from build123d import *

# Parameters (mm, degrees)
MAIN_BOARD_W          = 1000
MAIN_BOARD_H          = 750
MAINBOARD_DEPTH       = 20
CUT_EXTRUDE9_REACH    = 627.32
SKETCH5_R             = 10
SKETCH5_8_R           = 110
SKETCH5_8_R_2         = 105
CUT_EXTRUDE10_DEPTH   = 15
LPATTERN1_START       = 5
LPATTERN1_OUTLINE_R   = 110
LPATTERN1_OUTLINE_R_2 = 105
LPATTERN1_DEPTH       = 15


# Read off the part's stored shape, not the designer's step: LPattern1
with BuildPart() as part:
    # Main Board → MainBoard (new body)
    with BuildSketch(Plane(origin=(0, 0, 0), x_dir=(0, 0, -1), z_dir=(1, 0, 0))):
        Rectangle(MAIN_BOARD_W, MAIN_BOARD_H)
    extrude(amount=MAINBOARD_DEPTH)

    # Sketch5 → Cut-Extrude9 (cut, up to next)
    with BuildSketch(Plane(origin=(20, 0, 0), x_dir=(0, 0, -1), z_dir=(1, 0, 0)), mode=Mode.PRIVATE) as cut_extrude9_sk1:
        with Locations((-250, 125)):
            Circle(SKETCH5_R)
    cut_extrude9_tool1 = extrude(cut_extrude9_sk1.sketch, amount=-CUT_EXTRUDE9_REACH, mode=Mode.PRIVATE) & part.part
    add(cut_extrude9_tool1.solids().sort_by_distance((20, 125, 250))[0], mode=Mode.SUBTRACT)

    # Sketch5<8> → Cut-Extrude10 (cut)
    with BuildSketch(Plane(origin=(20, 0, 0), x_dir=(0, 0, -1), z_dir=(1, 0, 0))):
        with Locations((-250, 125)):
            Circle(SKETCH5_8_R)
        with Locations((-250, 125)):
            Circle(SKETCH5_8_R_2, mode=Mode.SUBTRACT)
    extrude(amount=-CUT_EXTRUDE10_DEPTH, mode=Mode.SUBTRACT)

    # LPattern1 outline → LPattern1 (cut)
    # profile 1 of 4: a face of its own
    with BuildSketch(Plane.YZ.offset(LPATTERN1_START)):
        with Locations((-91, 125)):
            Circle(LPATTERN1_OUTLINE_R)
        with Locations((-91, 125)):
            Circle(LPATTERN1_OUTLINE_R_2, mode=Mode.SUBTRACT)
    # profile 2 of 4: a face of its own
    with BuildSketch(Plane.YZ.offset(LPATTERN1_START)):
        with Locations((125, -250)):
            Circle(LPATTERN1_OUTLINE_R)
        with Locations((125, -250)):
            Circle(LPATTERN1_OUTLINE_R_2, mode=Mode.SUBTRACT)
    # profile 3 of 4: a face of its own
    with BuildSketch(Plane.YZ.offset(LPATTERN1_START)):
        with Locations((125, 0)):
            Circle(LPATTERN1_OUTLINE_R)
        with Locations((125, 0)):
            Circle(LPATTERN1_OUTLINE_R_2, mode=Mode.SUBTRACT)
    # profile 4 of 4: a face of its own
    with BuildSketch(Plane.YZ.offset(LPATTERN1_START)):
        with Locations((-91, -125)):
            Circle(LPATTERN1_OUTLINE_R)
        with Locations((-91, -125)):
            Circle(LPATTERN1_OUTLINE_R_2, mode=Mode.SUBTRACT)
    extrude(amount=LPATTERN1_DEPTH, mode=Mode.SUBTRACT)


solid = part.part
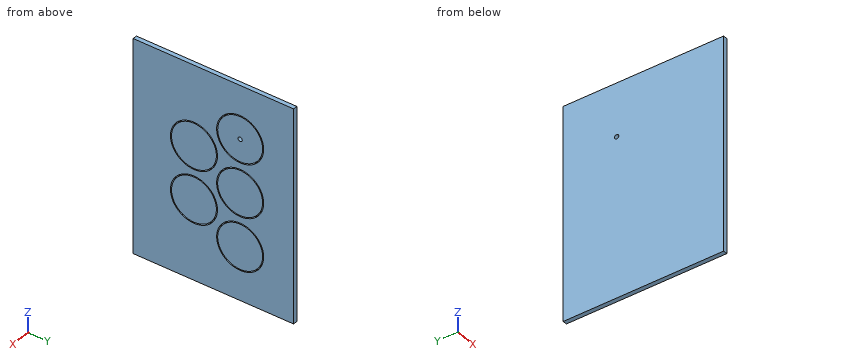
The listing builds one solid part. Answer for the finished solid, in the listing's coordinates (mm). Coordinates: 2 decimals unless noted, no trailing zeros. Write each loop counter-clockwise with the first axis right and the second up, starting at its lowest first coordinate (ties: lowest second). Pieces come first, ordered by that corner, then holes. Notation, with made-up numbers: (68, -30.5) -> (114, -30.5) arc R24 ccw to (114, -14.5) -> close; hole circle Ø2 at (3, 56). An arc over 180 degrees is marked (long way). One line per question, with ' | ' between items.
1. Section A-A (x = 14.25) is taken. State how many separate pieces and enclosed holes the cut face has, and give its area (3 significant figures).
Verdict:
separate pieces: 6 | enclosed holes: 6 | area: 733,000 mm^2
2. Straight lines are drawn through the part: line 1 (Y direction, x = 15.25, z = 250); line 2 (Z direction, x = 11.5, y = -91); line 3 (Y direction, x = 18.75, z = 219.5). For each, find the intervals that lie inside material, in ascending order.
Verdict:
line 1: y = -375 to 15, 20 to 115, 135 to 230, 235 to 375 | line 2: z = -500 to -235, -230 to -20, -15 to 15, 20 to 230, 235 to 500 | line 3: y = -375 to -147.3, -136.77 to -45.23, -34.7 to 19.31, 24.53 to 225.47, 230.69 to 375
3. Section C-C (z = -159) is taken. Determine the outline of the cut face in (x, y).
Verdict:
outline: (0, -375) -> (20, -375) -> (20, -195.61) -> (5, -195.61) -> (5, -190.34) -> (20, -190.34) -> (20, 8.34) -> (5, 8.34) -> (5, 13.61) -> (20, 13.61) -> (20, 63.2) -> (5, 63.2) -> (5, 72.62) -> (20, 72.62) -> (20, 177.38) -> (5, 177.38) -> (5, 186.8) -> (20, 186.8) -> (20, 375) -> (0, 375) -> close
4. Section B-B (y = -91) is taken. Determine the outline of the cut face in (x, z).
Verdict:
outline: (0, -500) -> (20, -500) -> (20, -235) -> (5, -235) -> (5, -230) -> (20, -230) -> (20, -20) -> (5, -20) -> (5, -15) -> (20, -15) -> (20, 15) -> (5, 15) -> (5, 20) -> (20, 20) -> (20, 230) -> (5, 230) -> (5, 235) -> (20, 235) -> (20, 500) -> (0, 500) -> close
